from build123d import *

# Parameters (mm, degrees)
CROQUIS1_R              = 2.5
SALIENTE_EXTRUIR1_DEPTH = 1.25
SALIENTE_EXTRUIR4_DEPTH = 2.5
CROQUIS6_R              = 12.575
CORTAR_EXTRUIR3_DEPTH   = 10
SALIENTE_EXTRUIR5_DEPTH = 200
CROQUIS8_R              = 12.575
SALIENTE_EXTRUIR6_DEPTH = 21
CROQUIS9_W              = 200
CROQUIS9_H              = 30.25
CROQUIS9_H_2            = 5
CROQUIS9_W_2            = 2
CORTAR_EXTRUIR6_DEPTH   = 133.67370689
CROQUIS10_W             = 23.5
CROQUIS10_H             = 5
SALIENTE_EXTRUIR7_DEPTH = 15
CROQUIS11_W             = 23.5
CROQUIS11_H             = 5
SALIENTE_EXTRUIR8_DEPTH = 15


with BuildPart() as part:
    # Croquis1 → Saliente-Extruir1 (new, symmetric)
    with BuildSketch(Plane(origin=(0, 0, 0), x_dir=(0, 0, -1), z_dir=(1, 0, 0))):
        with BuildLine():
            Line((125, -2.5), (-125, -2.5))
            Line((-125, -2.5), (-125, 2.5))
            Line((-125, 2.5), (-123, 2.5))
            Line((-123, 2.5), (-117, 17.5))
            ThreePointArc((-117, 17.5), (-110, 24.5), (-103, 17.5))
            Line((-103, 17.5), (-97, 2.5))
            Line((-97, 2.5), (125, 2.5))
            Line((125, 2.5), (125, -2.5))
        make_face()
        with Locations((-110, 17.5)):
            Circle(CROQUIS1_R, mode=Mode.SUBTRACT)
    extrude(amount=SALIENTE_EXTRUIR1_DEPTH, both=True)

    # Croquis5 → Saliente-Extruir4 (add, through all)
    with BuildSketch(Plane(origin=(1.25, 0, 0), x_dir=(0, 0, -1), z_dir=(1, 0, 0))):
        with BuildLine():
            ThreePointArc((-100, 10), (-110, 5), (-120, 10))
            Line((-120, 10), (-121.0552482, 7.361879501))
            ThreePointArc((-121.0552482, 7.361879501), (-110, 2.5), (-98.9447518, 7.361879501))
            Line((-98.9447518, 7.361879501), (-100, 10))
        make_face()
        with BuildLine():
            Line((-121.0552482, 7.361879501), (-120, 10))
            ThreePointArc((-120, 10), (-113.952847075, 29.358541226), (-97.5, 17.5))
            ThreePointArc((-97.5, 17.5), (-98.141458774, 13.547152925), (-100, 10))
            Line((-100, 10), (-98.9447518, 7.361879501))
            ThreePointArc((-98.9447518, 7.361879501), (-96.020931308, 12.060731804), (-95, 17.5))
            ThreePointArc((-95, 17.5), (-115.439268196, 31.479068692), (-121.0552482, 7.361879501))
        make_face()
    extrude(amount=-SALIENTE_EXTRUIR4_DEPTH)

    # Croquis6 → Cortar-Extruir3 (cut)
    with BuildSketch(Plane(origin=(1.25, 0, 0), x_dir=(0, 0, -1), z_dir=(1, 0, 0))):
        with Locations((-110, 17.5)):
            Circle(CROQUIS6_R)
    extrude(amount=-CORTAR_EXTRUIR3_DEPTH, mode=Mode.SUBTRACT)

    # Croquis7 → Saliente-Extruir5 (add)
    with BuildSketch(Plane(origin=(0, 0, -125), x_dir=(-1, 0, 0), z_dir=(0, 0, -1))):
        Polygon((3.75, 37.75), (3.75, -2.5), (1.25, -2.5), (1.25, 2.5), (1.25, 32.75), (-1.25, 32.75), (-1.25, 37.75), align=None)
    extrude(amount=-SALIENTE_EXTRUIR5_DEPTH)

    # Croquis8 → Saliente-Extruir6 (add)
    with BuildSketch(Plane.ZY.offset(1.25)):
        with BuildLine():
            Line((98.9447518, 7.361879501), (97, 2.5))
            Line((97, 2.5), (95, 2.5))
            Line((95, 2.5), (95, -2.5))
            Line((95, -2.5), (125, -2.5))
            Line((125, -2.5), (125, 2.5))
            Line((125, 2.5), (123, 2.5))
            Line((123, 2.5), (121.0552482, 7.361879501))
            ThreePointArc((121.0552482, 7.361879501), (110, 32.5), (98.9447518, 7.361879501))
        make_face()
        with Locations(Location((110, 17.5, 0), (0, 0, 180))):
            Circle(CROQUIS8_R, mode=Mode.SUBTRACT)
    extrude(amount=SALIENTE_EXTRUIR6_DEPTH)

    # Croquis9 → Cortar-Extruir6 (cut, through all)
    with BuildSketch(Plane(origin=(1.25, 0, 0), x_dir=(0, 0, -1), z_dir=(1, 0, 0))):
        Polygon((-75, 2.5), (-97, 2.5), (-97, -2.5), (125, -2.5), (125, 2.5), align=None)
        with Locations((25, 17.625)):
            Rectangle(CROQUIS9_W, CROQUIS9_H)
        with Locations((25, 35.25)):
            Rectangle(CROQUIS9_W, CROQUIS9_H_2)
        with Locations((-124, 0)):
            Rectangle(CROQUIS9_W_2, CROQUIS9_H_2)
    extrude(amount=-CORTAR_EXTRUIR6_DEPTH, mode=Mode.SUBTRACT)

    # Croquis10 → Saliente-Extruir7 (add)
    with BuildSketch(Plane(origin=(0, 0, 97), x_dir=(-1, 0, 0), z_dir=(0, 0, -1))):
        with Locations((10.5, 0)):
            Rectangle(CROQUIS10_W, CROQUIS10_H)
    extrude(amount=SALIENTE_EXTRUIR7_DEPTH)

    # Croquis11 → Saliente-Extruir8 (add)
    with BuildSketch(Plane.XY.offset(123)):
        with Locations((-10.5, 0)):
            Rectangle(CROQUIS11_W, CROQUIS11_H)
    extrude(amount=SALIENTE_EXTRUIR8_DEPTH)


solid = part.part
Could you check a few things on this model? Use its own coordinates, in mm. Coordinates: 2 decimals unless noted, no trailing zeros. Order: outer loops, then holes, each group sorted by start corner. A loop starts at its lowest first (then second) coordinate and runs counter-clockwise, first axis right, second up. Notation, with made-up numbers: (18.5, 29.5) -> (52.5, 29.5) arc R29 cw to (52.5, 57.5) -> close; hole circle Ø10 at (2, -14). An arc over 180 degrees is marked (long way). One line per item, written item: value. Start each with the question number.
1) If I drill on L1, parallel to Z at x = -12.75, y = 17.5 (3 decimals); L2, parallel to Y at x = -16.25, z = 110 (3 decimals); L3, parallel to Y at x = -11.75, z = 85.5, over which ranges is the centre line in solid material (lowest first)? Write a range as [from, to].
2) We'd pull the mould along Z, two halves only. Please class faces 1 (the flat face through (-11, 0, 138)), 2 (the flat face through (-11, -2.5, 110)), 3 (the flat face through (-10, 0, 82)), 4 (the cylindrical face through (-10.336, 13.723, 98.006)): +Z half, -Z half, draft (parallel to the pull), parting line (faces both ways), or undercut.
3) Imagine slicing it at B-B on z = 110. List the corners of the cut face in (x, y) for me (3 decimals), plus the area to 3 significant figures.
4) Imagine slicing it at D-D on z = 118.5. List the corners of the cut face in (x, y) for me.
5) I'm going to push flat-ended pins straight in: pin 1 (12 mm diameter, centred on x = -6.5, y = 24, fed in from -Z); pin 2 (4.5 mm diameter, centred on x = -10.5, z = 91, fed in from +Y); pin 3 (8 mm diameter, centred on x = -18.5, z = 96, fed in from +Y). Where does each tip first touch, or does it pass through?
6) Imagine slicing it at A-A on x = -6.75. List the corners of the cut face in (y, z) for me (3 decimals), plus the area to 3 significant figures.
7) Imagine slicing it at C-C on y = 27.5. List the corners of the cut face in (x, z) for me, plus the area to 3 significant figures.
Answer list:
1. L1: z = [95, 97.425], [122.575, 125]
1. L2: y = [-2.5, 4.925], [30.075, 32.5]
1. L3: y = [-2.5, 2.5]
2. face 1: +Z half
2. face 2: draft
2. face 3: -Z half
2. face 4: undercut
3. outline: (-22.25, -2.5) -> (1.25, -2.5) -> (1.25, 4.925) -> (-22.25, 4.925) -> close; (-22.25, 30.075) -> (1.25, 30.075) -> (1.25, 32.5) -> (-22.25, 32.5) -> close
3. area: 231 mm2
4. outline: (-22.25, -2.5) -> (1.25, -2.5) -> (1.25, 8.23) -> (-22.25, 8.23) -> close; (-22.25, 26.77) -> (1.25, 26.77) -> (1.25, 29.86) -> (-22.25, 29.86) -> close
5. pin 1: stops at z = 95.01
5. pin 2: stops at y = 2.5
5. pin 3: stops at y = 28.68
6. outline: (-2.5, 82) -> (2.5, 82) -> (2.5, 97) -> (7.362, 98.945) arc R15 ccw (long way) to (7.362, 121.055) -> (2.5, 123) -> (2.5, 138) -> (-2.5, 138) -> close; hole circle Ø25.15 at (17.5, 110)
6. area: 533 mm2
7. outline: (-22.25, 98.82) -> (1.25, 98.82) -> (1.25, 102.38) -> (-22.25, 102.38) -> close; (-22.25, 117.62) -> (1.25, 117.62) -> (1.25, 121.18) -> (-22.25, 121.18) -> close
7. area: 167 mm2
